Design review of the part built by this model. Coordinates are the model's own, in mm. A direction names the side the tool comes from. Give positions to 0.01 mm unless a question says otherwise; leave off trailing zeros. Order: outer loops, then holes, each group sorted by start corner. A loop starts at its lowest first (then second) coordinate and runs counter-clockwise, first axis right, second up. Notation, with made-up numbers: (-35, 36) -> (-16, 36) arc R26 cw to (-16, 63) -> close; hole circle Ø2 at (45.5, 22.5). An arc over 180 degrees is marked (long way). Use a Markdown table: item, result. Add a question column.
```python
from build123d import *

# Parameters (mm, degrees)
BOSS_EXTRUDE1_DEPTH     = 6.35
M5_CLEARANCE_HOLE1_D    = 5.3
SKETCH5_R               = 10
CUT_EXTRUDE1_DEPTH      = 124.856055565
F_3_8_CLEARANCE_HOLE1_D = 9.8044
FILLET1_R               = 120
FILLET2_R               = 5


with BuildPart() as part:
    # Sketch1 → Boss-Extrude1 (new body)
    with BuildSketch(Plane(origin=(0, 0, 0), x_dir=(1, 0, 0), z_dir=(0, 1, 0))):
        with BuildLine():
            Line((-12.7, -120), (12.7, -120))
            Line((12.7, -120), (12.7, -27.179220004))
            ThreePointArc((12.7, -27.179220004), (0, 30), (-12.7, -27.179220004))
            Line((-12.7, -27.179220004), (-12.7, -120))
        make_face()
    extrude(amount=BOSS_EXTRUDE1_DEPTH)

    # M5 Clearance Hole1 (through all)
    with Locations(Plane(origin=(0, 0, 0), x_dir=(-1, 0, 0), z_dir=(0, -1, 0))):
        with Locations((0, 17.5), (12.374368671, 12.374368671), (17.5, 0), (12.374368671, -12.374368671), (0, -17.5), (-12.374368671, -12.374368671), (-17.5, 0), (-12.374368671, 12.374368671)):
            Hole(M5_CLEARANCE_HOLE1_D / 2)

    # Sketch5 → Cut-Extrude1 (cut, through all)
    with BuildSketch(Plane.XZ):
        with Locations(Location((0, 0, 0), (0, 0, 270))):
            Circle(SKETCH5_R)
    extrude(amount=-CUT_EXTRUDE1_DEPTH, mode=Mode.SUBTRACT)

    # 3_8 Clearance Hole1 (through all)
    with Locations(Plane(origin=(0, 0, 0), x_dir=(-1, 0, 0), z_dir=(0, -1, 0))):
        with Locations((0, -85), (0, -110)):
            Hole(F_3_8_CLEARANCE_HOLE1_D / 2)

    # Fillet1
    fillet1_edges = [part.edges().sort_by_distance(p)[0] for p in [
        (-12.7, 3.175, 27.179220004),
        (12.7, 3.175, 27.179220004),
    ]]
    fillet(fillet1_edges, radius=FILLET1_R)

    # Fillet2
    fillet2_edges = [part.edges().sort_by_distance(p)[0] for p in [
        (12.7, 3.175, 120),
        (-12.7, 3.175, 120),
    ]]
    fillet(fillet2_edges, radius=FILLET2_R)


solid = part.part
```
1) Add section A-A (z = 0). Give the boundary of the cut face in (x, y).
2) Insertion check: pin 1 (1.5 mm diameter, centred on x = 9.5, y = 2.5, fed in from -Z); pin 2 (1 mm diameter, centred on y = 2, z = 16, fed in from -X); pin 3 (4 mm diameter, centred on x = -12.37, z = -12.37, fed in from +Y); pin 4 (1.5 mm diameter, centred on x = -21.5, y = 1, fed in from -Z). Each pin has a flat end and moves straight along its axis. Give the tip position at first contact, or say it passes through.
3) Add section D-D (z = 22.5). Give the boundary of the cut face in (x, y), then the cut area to 3 significant figures.
4) Add section B-B (z = 110). Give the boundary of the cut face in (x, y), then the cut area to 3 significant figures.
5) For L1, parallel to X at y = 0.75, z = 85; L2, parallel to Z at x = -4, y = 2; L3, parallel to X at y = 4.25, z = 17.5, list the stretches that pass through material, from the lowest coordinate up. Write a range as [from, to].
6) Machinability: for faces 5 (the flat face through (-12.7, 3, 92)), 6 (the cylindrical face through (14.902, 3.219, 11.578)), which of the approach directions +Z, -Z, +X, -X, +Y, -Y give a long, thin tool a straight path to every point of the face, cutting with its end or side? Answer none if there is none.
7) The part is to be moulded in two halves that separate along X. For faces 1 (the cylindrical face through (-11.27, 3.22, 118.5)), 2 (the cylindrical face through (0.863, 3.131, -29.988)), 3 (the flat face through (12.7, 3, 93)), 4 (the cylindrical face through (-1.063, 3.219, 89.786)), say which applies: +X half, -X half, draft (parallel to the pull), parting line (faces both ways), or undercut.
8) Add section C-C (x = -17.5). Give the boundary of the cut face in (y, z), then the cut area to 3 significant figures.
Worked answers:
| question | item | result |
|---|---|---|
| 1 | outline | (-30, 0) -> (-20.15, 0) -> (-20.15, 6.35) -> (-30, 6.35) -> close; (-14.85, 0) -> (-10, 0) -> (-10, 6.35) -> (-14.85, 6.35) -> close; (10, 0) -> (14.85, 0) -> (14.85, 6.35) -> (10, 6.35) -> close; (20.15, 0) -> (30, 0) -> (30, 6.35) -> (20.15, 6.35) -> close |
| 2 | pin 1 | z = -28.7 |
| 2 | pin 2 | x = -25.76 |
| 2 | pin 3 | through |
| 2 | pin 4 | z = -21.67 |
| 3 | outline | (-22.47, 0) -> (22.47, 0) -> (22.47, 6.35) -> (-22.47, 6.35) -> close |
| 3 | area | 285 mm^2 |
| 4 | outline | (-12.7, 0) -> (-4.9, 0) -> (-4.9, 6.35) -> (-12.7, 6.35) -> close; (4.9, 0) -> (12.7, 0) -> (12.7, 6.35) -> (4.9, 6.35) -> close |
| 4 | area | 99.0 mm^2 |
| 5 | L1 | [-12.7, -4.9], [4.9, 12.7] |
| 5 | L2 | [-29.73, -9.17], [9.17, 82.17], [87.83, 107.17], [112.83, 120] |
| 5 | L3 | [-24.76, -2.65], [2.65, 24.76] |
| 6 | face 5 | +Z, -X, +Y, -Y |
| 6 | face 6 | +Y, -Y |
| 7 | face 1 | -X half |
| 7 | face 2 | parting line |
| 7 | face 3 | +X half |
| 7 | face 4 | undercut |
| 8 | outline | (0, -24.37) -> (6.35, -24.37) -> (6.35, -2.65) -> (0, -2.65) -> close; (0, 2.65) -> (6.35, 2.65) -> (6.35, 36.33) -> (0, 36.33) -> close |
| 8 | area | 352 mm^2 |
